from build123d import *

# Parameters (mm, degrees)
SKETCH1_W           = 25.4
SKETCH1_H           = 44.45
SKETCH1_W_2         = 19.05
SKETCH1_H_2         = 19.05
BOSS_EXTRUDE1_DEPTH = 3.175
SKETCH4_W           = 3.175
SKETCH4_H           = 44.45
BOSS_EXTRUDE3_DEPTH = 5.08
MOVE_FACE1_BY       = 0.508


with BuildPart() as part:
    # Sketch1 → Boss-Extrude1 (new body)
    with BuildSketch(Plane.XY):
        Rectangle(SKETCH1_W, SKETCH1_H)
        Rectangle(SKETCH1_W_2, SKETCH1_H_2, mode=Mode.SUBTRACT)
    extrude(amount=BOSS_EXTRUDE1_DEPTH)

    # Sketch4 → Boss-Extrude3 (add)
    with BuildSketch(Plane.ZY.offset(12.7)):
        with Locations((1.5875, 0)):
            Rectangle(SKETCH4_W, SKETCH4_H)
    extrude(amount=BOSS_EXTRUDE3_DEPTH)

    # Move Face1: a face moved inward by 0.508
    extrude(part.faces().sort_by_distance((-2.54, -11.1125, 3.175))[0], amount=MOVE_FACE1_BY, dir=(0, 0, -1), mode=Mode.SUBTRACT)


solid = part.part
Model file for the job. Use its own axes, mm. A direction names the side the tool comes from. Give positions to 0.01 mm unless a question says otherwise; leave off trailing zeros. Order: outer loops, then holes, each group sorted by start corner. A loop starts at its lowest first (then second) coordinate and runs counter-clockwise, first axis right, second up. Notation, with made-up numbers: M -15,81 L 37,81 A35 ccw 37,117 Z; hole C 5.5,69 d7. An arc over 180 degrees is marked long. Put each result on its own line as item: value. Start each with the question number.
(1) Drill centre lines: L1, parallel to X at y = -6, z = 1.1 (3 decimals); L2, parallel to Y at x = -2.5, z = 1.7 (3 decimals). Where is each one in solid material? Low to high. Write a range as [from, to].
(2) Tool access for faces 5 (the face through (0, -9.525, 1)), 6 (the face through (-12, 0, 0)): list every direction of +Z, -Z, +X, -X, +Y, -Y with a clear straight run to the whole face (end or side of a thin tool).
(3) Band-saw the part on B-B on x = 8.5. Give the cut face in (y, z) (3 decimals), then the cut area to 3 significant figures.
(4) Pull direction Y, two halves, no side cores. Call faces 1 (the face through (-17.78, 0, 1)), 2 (the face through (-2, -22.225, 1)), 3 (the face through (0, 9.525, 1)), 4 (the face through (-2, 22.225, 1)): released by +Y, released by -Y, zero draft, split by the parting line, or undercut.
(5) Band-saw the part on C-C on z = 0.7. Give the cut face in (x, y) (3 decimals), then the cut area to 3 significant figures.
(6) Band-saw the part on A-A on y = -1. Give the cut face in (x, z) (3 decimals).
Results below:
1. L1: x = [-17.78, -9.525], [9.525, 12.7]
1. L2: y = [-22.225, -9.525], [9.525, 22.225]
2. face 5: +Z, -Z
2. face 6: -Z, +X, -X, +Y, -Y
3. outline: M -22.225,0 L -9.525,0 L -9.525,2.667 L -22.225,2.667 Z; M 9.525,0 L 22.225,0 L 22.225,2.667 L 9.525,2.667 Z
3. area: 67.7 mm2
4. face 1: zero draft
4. face 2: released by -Y
4. face 3: undercut
4. face 4: released by +Y
5. outline: M -17.78,-22.225 L 12.7,-22.225 L 12.7,22.225 L -17.78,22.225 Z; hole M -9.525,-9.525 L 9.525,-9.525 L 9.525,9.525 L -9.525,9.525 Z
5. area: 992 mm2
6. outline: M -17.78,0 L -9.525,0 L -9.525,2.667 L -17.78,2.667 Z; M 9.525,0 L 12.7,0 L 12.7,2.667 L 9.525,2.667 Z
